Model file for the job. Use its own axes, mm. A direction names the side the tool comes from. Round coordinates to 2 decimals unless told otherwise and drop trailing zeros. Loops run counter-clockwise (first coordinate to the right, second up) from the corner with the lowest first, then second, coordinate; pieces in that order, holes last. Notation, with made-up numbers: M -9,72 L 35,72 A19 cw 35,105 Z; hole C 67,47 d9. An arc over 180 degrees is marked long. Use a Markdown table: item, result. Add a question column.
Item 1: Wall check: L1, parallel to Y at x = 115.05, z = 82; L2, parallel to X at y = -8.5, z = 67; L3, parallel to X at y = 6, z = 104. Give the ranges that are in metal, low to high. Write a range as from..to.
Item 2: Saw through at B-B on z = 0. Write the cut outline in (x, y).
Item 3: Two-plate mould, pull along Z, no slides. Class faces 1 (the flat face through (-113.5, 0, 82)), 2 (the flat face through (-1, 0, 100)), 3 (the flat face through (-19, 47, -52)): +Z half, -Z half, draft (parallel to the pull), parting line (faces both ways), or undercut.
Item 4: Tool access for faces 4 (the flat face through (-1, 35.5, 85)), 5 (the flat face through (113.5, 0, 82)), 6 (the flat face through (1, 44, 1)): list every direction of +Z, -Z, +X, -X, +Y, -Y with a clear straight run to the whole face (end or side of a thin tool).
Item 5: Saw through at D-D on y = -15. Give the number of separate pieces and of enclosed holes in the cut face, then the cut area to 3 significant figures.
Item 6: Pin check, flat tips, straight feed: P1, Ø1, axis at x = 68, y = -33.5, coming from the +Z side; P2, Ø6, axis at x = -0.5, y = -16.5, coming from the +Z side; P3, Ø8, axis at x = 81.5, z = 68, coming from the +Y side. Stop position of each tip, or through.
Item 7: Saw through at C-C on z = 105.5. Write the cut outline in (x, y).
Item 8: Saw through at A-A on x = 0. Write the cut outline in (y, z).
```python
from build123d import *

# Parameters (mm, degrees)
F0_R      = 80
F1_DEPTH  = 47
F2_W      = 130
F2_H      = 71
F3_DEPTH  = 100
F4_W      = 79.5
F4_H      = 10
F6_R      = 10
F7_R      = 80
F8_DEPTH  = 47
F9_R      = 55
F10_DEPTH = 3


# Not quite as in the source:
# - a pattern or mirror of a feature is missing from the dataset's text; its kind, count and spacing are read off the source's solid


with BuildPart() as f1:
    # F0 (on Front) → F1 (new body)
    with BuildSketch(Plane.XZ):
        Circle(F0_R)
    extrude(amount=F1_DEPTH)

    # F2 (on Top) → F3 (join)
    with BuildSketch(Plane.XY):
        Rectangle(F2_W, F2_H)
    extrude(amount=F3_DEPTH)

    # F4 (on Front) → F5 (revolve)
    with BuildSketch(Plane.XZ):
        Polygon((79.5, 114.5), (79.5, 92), (79.5, 82), (113.5, 82), (113.5, 114.5), (116.5, 114.5), (116.5, 117.5), (98, 117.5), (98, 114.5), align=None)
        with Locations((39.75, 87)):
            Rectangle(F4_W, F4_H)
    f5 = revolve(axis=Axis((96.5, 0, 82), (-1, 0, 0)))

    # F5_copies: F5 across plane
    add(f5.mirror(Plane(origin=(0, 0, 0), x_dir=(0, 0, -1), z_dir=(-1, 0, 0))))

    # F6
    f6_edges = [f1.edges().sort_by_distance(p)[0] for p in [
        (79.5, 0, 72),
        (-79.5, 0, 72),
    ]]
    fillet(f6_edges, radius=F6_R)

    # F7 (on Front) → F8 (join)
    with BuildSketch(Plane.XZ):
        Circle(F7_R)
    extrude(amount=-F8_DEPTH)

    # F9 (on face) → F10 (cut)
    with BuildSketch(Plane(origin=(0, 47, 0), x_dir=(-1, 0, 0), z_dir=(0, 1, 0))):
        Circle(F9_R)
    extrude(amount=-F10_DEPTH, mode=Mode.SUBTRACT)


solid = f1.part
```
Entries:
| question | item | result |
|---|---|---|
| 1 | L1 | -35.5..-32.5, 32.5..35.5 |
| 1 | L2 | -113.5..-79.11, -65..65, 79.11..113.5 |
| 1 | L3 | -113.5..-79.5, 79.5..113.5 |
| 2 | outline | M -80,-47 L 80,-47 L 80,47 L 55,47 L 55,44 L -55,44 L -55,47 L -80,47 Z |
| 3 | face 1 | undercut |
| 3 | face 2 | +Z half |
| 3 | face 3 | draft |
| 4 | face 4 | +Z, +Y |
| 4 | face 5 | +X |
| 4 | face 6 | +Y |
| 5 | separate pieces | 3 |
| 5 | enclosed holes | 0 |
| 5 | area | 28,200 mm2 |
| 6 | P1 | z = 42.94 |
| 6 | P2 | z = 100 |
| 6 | P3 | y = 30.92 |
| 7 | outline | M -116.5,-26.61 L -98,-26.61 L -98,-22.45 L -79.5,-22.45 L -79.5,22.45 L -98,22.45 L -98,26.61 L -116.5,26.61 L -116.5,22.45 L -113.5,22.45 L -113.5,-22.45 L -116.5,-22.45 Z; M 79.5,-22.45 L 98,-22.45 L 98,-26.61 L 116.5,-26.61 L 116.5,-22.45 L 113.5,-22.45 L 113.5,22.45 L 116.5,22.45 L 116.5,26.61 L 98,26.61 L 98,22.45 L 79.5,22.45 Z |
| 8 | outline | M -47,-80 L 47,-80 L 47,-55 L 44,-55 L 44,55 L 47,55 L 47,80 L 35.5,80 L 35.5,100 L -35.5,100 L -35.5,80 L -47,80 Z |
